```python
from build123d import *

# Parameters (mm, degrees)
SKETCH1_R           = 3.7
SKETCH1_R_2         = 3.1
SKETCH1_R_3         = 2.4
BOSS_EXTRUDE2_DEPTH = 7.84
SKETCH1_5_R         = 3.1
SKETCH1_5_R_2       = 2.4
CUT_EXTRUDE1_DEPTH  = 1
SKETCH3_R           = 3.1
SKETCH3_R_2         = 2.4
CUT_EXTRUDE2_DEPTH  = 1
BOSS_EXTRUDE3_DEPTH = 7.84
CUT_EXTRUDE3_REACH  = 17.91
CUT_EXTRUDE4_DEPTH  = 16.90960716
SKETCH4_5_R         = 2.7
BOSS_EXTRUDE4_DEPTH = 7.4
CUT_EXTRUDE5_DEPTH  = 15.561785605


with BuildPart() as part:
    # Sketch1 → Boss-Extrude2 (new body)
    with BuildSketch(Plane(origin=(0, 0, 0), x_dir=(1, 0, 0), z_dir=(0, 1, 0))):
        with Locations(Location((0, 0, 0), (0, 0, 270))):
            Circle(SKETCH1_R)
        Circle(SKETCH1_R_2, mode=Mode.SUBTRACT)
        Circle(SKETCH1_R_2)
        with Locations(Location((0, 0, 0), (0, 0, 270))):
            Circle(SKETCH1_R_3, mode=Mode.SUBTRACT)
    extrude(amount=BOSS_EXTRUDE2_DEPTH)

    # Sketch1<5> → Cut-Extrude1 (cut)
    with BuildSketch(Plane(origin=(0, 0, 0), x_dir=(1, 0, 0), z_dir=(0, 1, 0))):
        with Locations(Location((0, 0, 0), (0, 0, 270))):
            Circle(SKETCH1_5_R)
        with Locations(Location((0, 0, 0), (0, 0, 270))):
            Circle(SKETCH1_5_R_2, mode=Mode.SUBTRACT)
    extrude(amount=CUT_EXTRUDE1_DEPTH, mode=Mode.SUBTRACT)

    # Sketch3 → Cut-Extrude2 (cut)
    with BuildSketch(Plane(origin=(0, 7.84, 0), x_dir=(1, 0, 0), z_dir=(0, 1, 0))):
        with Locations(Location((0, 0, 0), (0, 0, 270))):
            Circle(SKETCH3_R)
        with Locations(Location((0, 0, 0), (0, 0, 270))):
            Circle(SKETCH3_R_2, mode=Mode.SUBTRACT)
    extrude(amount=-CUT_EXTRUDE2_DEPTH, mode=Mode.SUBTRACT)

    # Sketch1<6> → Boss-Extrude3 (add)
    with BuildSketch(Plane(origin=(0, 0, 0), x_dir=(1, 0, 0), z_dir=(0, 1, 0))):
        with BuildLine():
            Line((-11.7, -2.7), (-11.7, -3.7))
            Line((-11.7, -3.7), (0, -3.7))
            ThreePointArc((0, -3.7), (-1.360147051, -3.440930107), (-2.529822128, -2.7))
            Line((-2.529822128, -2.7), (-11.7, -2.7))
        make_face()
        with BuildLine():
            Line((-11.7, 3.7), (-11.7, 2.7))
            Line((-11.7, 2.7), (-2.529822128, 2.7))
            ThreePointArc((-2.529822128, 2.7), (-1.360147051, 3.440930107), (0, 3.7))
            Line((0, 3.7), (-11.7, 3.7))
        make_face()
    extrude(amount=BOSS_EXTRUDE3_DEPTH)

    # Cut-Extrude3: up to this face of the body (flat: up to its plane)
    cut_extrude3_end = Plane(part.part.faces().sort_by_distance((-5.85, 3.92, 3.7))[0])
    # Sketch4 → Cut-Extrude3 (cut, up to the picked face)
    with BuildSketch(Plane(origin=(0, 0, -3.7), x_dir=(-1, 0, 0), z_dir=(0, 0, -1)), mode=Mode.PRIVATE) as cut_extrude3_sk1:
        with BuildLine():
            Line((11.7, 7.84), (7.78, 7.84))
            ThreePointArc((7.78, 7.84), (10.551858582, 6.691858582), (11.7, 3.92))
            Line((11.7, 3.92), (11.7, 7.84))
        make_face()
    cut_extrude3_tool1 = split(extrude(cut_extrude3_sk1.sketch, amount=-CUT_EXTRUDE3_REACH, mode=Mode.PRIVATE), bisect_by=cut_extrude3_end, keep=Keep.BOTH, mode=Mode.PRIVATE)
    # Sketch4 → Cut-Extrude3 (cut, up to the picked face)
    with BuildSketch(Plane(origin=(0, 0, -3.7), x_dir=(-1, 0, 0), z_dir=(0, 0, -1)), mode=Mode.PRIVATE) as cut_extrude3_sk2:
        with BuildLine():
            Line((11.7, 0), (11.7, 3.92))
            ThreePointArc((11.7, 3.92), (10.551858582, 1.148141418), (7.78, 0))
            Line((7.78, 0), (11.7, 0))
        make_face()
    cut_extrude3_tool2 = split(extrude(cut_extrude3_sk2.sketch, amount=-CUT_EXTRUDE3_REACH, mode=Mode.PRIVATE), bisect_by=cut_extrude3_end, keep=Keep.BOTH, mode=Mode.PRIVATE)
    add(cut_extrude3_tool1.solids().sort_by(Axis((-10.824398, 6.964398, -3.7), (0, 0, 1)))[0], mode=Mode.SUBTRACT)
    add(cut_extrude3_tool2.solids().sort_by(Axis((-10.824398, 0.875602, -3.7), (0, 0, 1)))[0], mode=Mode.SUBTRACT)

    # Sketch4<4> → Cut-Extrude4 (cut, through all)
    with BuildSketch(Plane(origin=(0, 0, -3.7), x_dir=(-1, 0, 0), z_dir=(0, 0, -1))):
        Polygon((8.78, 4.92), (8.78, 6.32), (6.78, 6.32), (6.78, 4.92), (5.38, 4.92), (5.38, 2.92), (6.78, 2.92), (6.78, 1.52), (8.78, 1.52), (8.78, 2.92), (10.18, 2.92), (10.18, 4.92), align=None)
    extrude(amount=-CUT_EXTRUDE4_DEPTH, mode=Mode.SUBTRACT)

    # Sketch4<5> → Boss-Extrude4 (add, through all)
    with BuildSketch(Plane(origin=(0, 0, -3.7), x_dir=(-1, 0, 0), z_dir=(0, 0, -1))):
        with Locations((7.78, 3.92)):
            Circle(SKETCH4_5_R)
        Polygon((8.78, 6.32), (8.78, 4.92), (10.18, 4.92), (10.18, 2.92), (8.78, 2.92), (8.78, 1.52), (6.78, 1.52), (6.78, 2.92), (5.38, 2.92), (5.38, 4.92), (6.78, 4.92), (6.78, 6.32), align=None, mode=Mode.SUBTRACT)
    extrude(amount=-BOSS_EXTRUDE4_DEPTH)

    # Sketch5 → Cut-Extrude5 (cut, through all)
    with BuildSketch(Plane(origin=(0, 0, 0), x_dir=(1, 0, 0), z_dir=(0, 1, 0))):
        with BuildLine():
            Line((-8.33, -2.15), (-8.33, 2.15))
            ThreePointArc((-8.33, 2.15), (-7.78, 2.7), (-7.23, 2.15))
            Line((-7.23, 2.15), (-7.23, -2.15))
            ThreePointArc((-7.23, -2.15), (-7.78, -2.7), (-8.33, -2.15))
        make_face()
    extrude(amount=CUT_EXTRUDE5_DEPTH, mode=Mode.SUBTRACT)


solid = part.part
```
For this review, take the finished solid that the model builds, in its own axes (mm). A direction names the side the tool comes from. Coordinates: 2 decimals unless noted, no trailing zeros. Write each loop counter-clockwise with the first axis right and the second up, starting at its lowest first coordinate (ties: lowest second). Pieces come first, ordered by that corner, then holes. Notation, with made-up numbers: (39.25, 32.25) -> (92.25, 32.25) arc R26 cw to (92.25, 54.25) -> close; hole circle Ø9 at (78, 23.5). An arc over 180 degrees is marked (long way). Put each result on its own line as item: value.
Q1. Tool access review of faces 5 (the flat face through (-5, 3, -2.7)), 6 (the flat face through (-5.38, 4, 0)), 7 (the cylindrical face through (0.931, 0.493, 2.957)): name each direction out of +Z, -Z, +X, -X, +Y, -Y from which nothing blocks a thin tool from reaching the whole face with its end or side.
From the geometry:
face 5: none
face 6: +Z, -Z
face 7: -Y
Q2. Clearance check with flat-ended pins moving along their axes: pin 1 Ø0.7 at (x, z) = (-6.5, 1) entering from +Y; pin 2 Ø1.5 at (x, z) = (-5, -0.5) entering from -Y; pin 3 Ø1.5 at (x, z) = (-9.5, -2.5) entering from +Y; pin 4 Ø3.5 at (x, z) = (0, 0) entering from -Y. State where each tip first meets the part, or that it passes through.
From the geometry:
pin 1: stops at y = 6.45
pin 2: stops at y = 2.14
pin 3: stops at y = 7.71
pin 4: passes through
Q3. Take a section at D-D, the plane y = 7. State the section outline as (x, z) points, then the cut area to 3 significant figures.
From the geometry:
outline: (-10.2, -3.7) -> (0, -3.7) arc R3.7 ccw to (0, 3.7) -> (-10.2, 3.7) -> (-10.2, 2.7) -> (-2.53, 2.7) arc R3.7 ccw to (-2.53, -2.7) -> (-10.2, -2.7) -> close; hole circle Ø6.2 at (0, 0)
area: 29.8 mm2
Q4. Take a section at A-A, the plane y = 5.5. State the section outline as (x, z) points, then the cut area to 3 significant figures.
From the geometry:
outline: (-11.37, -3.7) -> (-8.78, -3.7) -> (-8.78, 3.7) -> (-11.37, 3.7) -> (-11.37, 2.7) -> (-9.97, 2.7) -> (-9.97, -2.7) -> (-11.37, -2.7) -> close; (-6.78, -3.7) -> (0, -3.7) arc R3.7 ccw to (0, 3.7) -> (-6.78, 3.7) -> close; hole (-5.59, -2.7) -> (-2.53, -2.7) arc R3.7 cw to (-2.53, 2.7) -> (-5.59, 2.7) -> close; hole circle Ø4.8 at (0, 0)
area: 53.0 mm2
Q5. Take a section at C-C, the plane z = 0. Count the separate pieces of the cut face and the enclosed holes in it, then the cut area to 3 significant figures.
From the geometry:
separate pieces: 4
enclosed holes: 0
area: 24.7 mm2
Q6. Wall thickness on L1, parallel to Z at x = -7.75, y = 7.25; L2, parallel to X at y = 4, z = 0; L3, parallel to Z at x = -3, y = 5.25: over which ranges is each line inside the solid? List them lowest first.
From the geometry:
L1: z = -3.7 to -2.7, 2.7 to 3.7
L2: x = -10.48 to -10.18, -5.38 to -5.08, -3.7 to -2.4, 2.4 to 3.7
L3: z = -3.7 to -2.7, -2.17 to 2.17, 2.7 to 3.7
Q7. Take a section at B-B, the plane x = 1.75. State the section outline as (y, z) points, then the cut area to 3 significant figures.
From the geometry:
outline: (0, -3.26) -> (7.84, -3.26) -> (7.84, -2.56) -> (6.84, -2.56) -> (6.84, -1.64) -> (1, -1.64) -> (1, -2.56) -> (0, -2.56) -> close; (0, 2.56) -> (1, 2.56) -> (1, 1.64) -> (6.84, 1.64) -> (6.84, 2.56) -> (7.84, 2.56) -> (7.84, 3.26) -> (0, 3.26) -> close
area: 21.7 mm2
Q8. The part is to be moulded in two halves that separate along Y. For faces 1 (the flat face through (-5, 4, 3.7)), 2 (the flat face through (-3.3, 0, 0)), 3 (the flat face through (-6.78, 2, 0)), 4 (the flat face through (-8.78, 2, 0)), say which applies: +Y half, -Y half, draft (parallel to the pull), parting line (faces both ways), or undercut.
From the geometry:
face 1: draft
face 2: -Y half
face 3: undercut
face 4: undercut
